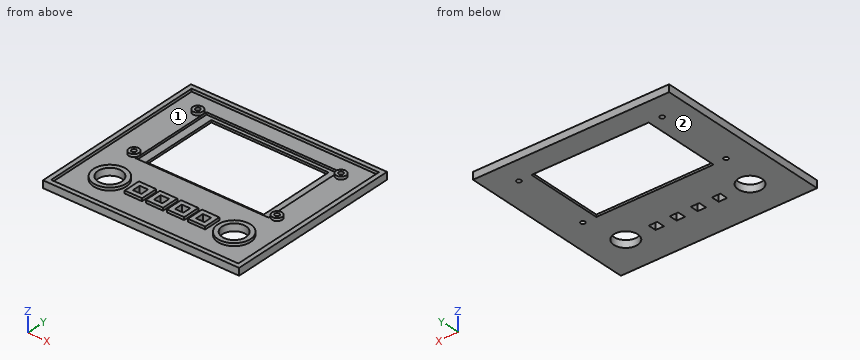
```python
from build123d import *

# Parameters (mm, degrees)
SKETCH1_W           = 139.7
SKETCH1_H           = 127
SKETCH1_R           = 8.5
SKETCH1_W_2         = 6
SKETCH1_H_2         = 5.8
SKETCH1_W_3         = 83.52
SKETCH1_H_3         = 55.68
BOSS_EXTRUDE1_DEPTH = 5.1375
SKETCH2_W           = 94.57
SKETCH2_H           = 60.88
SKETCH2_W_2         = 83.52
SKETCH2_H_2         = 55.68
CUT_EXTRUDE1_DEPTH  = 3.55
SKETCH3_R           = 1.6
SKETCH3_R_2         = 1.6002
CUT_EXTRUDE2_DEPTH  = 10
SKETCH4_W           = 133.35
SKETCH4_H           = 120.65
SKETCH4_R           = 3.6
SKETCH4_R_2         = 3.6002
SKETCH4_R_3         = 11.675
SKETCH4_W_2         = 12.35
SKETCH4_H_2         = 12.15
SKETCH4_W_3         = 94.57
SKETCH4_H_3         = 60.88
CUT_EXTRUDE3_DEPTH  = 1.9625


with BuildPart() as part:
    # Sketch1 → Boss-Extrude1 (new body)
    with BuildSketch(Plane.XY):
        with Locations((-0.265452364, -19.000597583)):
            Rectangle(SKETCH1_W, SKETCH1_H)
        with Locations((44.004207636, -55.869967583)):
            Circle(SKETCH1_R, mode=Mode.SUBTRACT)
        with Locations((-44.535112364, -55.869967583)):
            Circle(SKETCH1_R, mode=Mode.SUBTRACT)
        with Locations((-7.765452364, -55.869967583)):
            Rectangle(SKETCH1_W_2, SKETCH1_H_2, mode=Mode.SUBTRACT)
        Rectangle(SKETCH1_W_3, SKETCH1_H_3, mode=Mode.SUBTRACT)
        with Locations((-22.765452364, -55.869967583)):
            Rectangle(SKETCH1_W_2, SKETCH1_H_2, mode=Mode.SUBTRACT)
        with Locations((7.234547636, -55.869967583)):
            Rectangle(SKETCH1_W_2, SKETCH1_H_2, mode=Mode.SUBTRACT)
        with Locations((22.234547636, -55.869967583)):
            Rectangle(SKETCH1_W_2, SKETCH1_H_2, mode=Mode.SUBTRACT)
    extrude(amount=BOSS_EXTRUDE1_DEPTH)

    # Sketch2 → Cut-Extrude1 (cut)
    with BuildSketch(Plane.XY.offset(5.1375)):
        Rectangle(SKETCH2_W, SKETCH2_H)
        Rectangle(SKETCH2_W_2, SKETCH2_H_2, mode=Mode.SUBTRACT)
    extrude(amount=-CUT_EXTRUDE1_DEPTH, mode=Mode.SUBTRACT)

    # Sketch3 → Cut-Extrude2 (cut)
    with BuildSketch(Plane.XY.offset(5.1375)):
        with Locations((51.005027636, -27.450347583)):
            Circle(SKETCH3_R)
        with Locations((-51.034972364, 27.449652417)):
            Circle(SKETCH3_R)
        with Locations((51.005027636, 27.449652417)):
            Circle(SKETCH3_R)
        with Locations((-51.034972364, -27.449907583)):
            Circle(SKETCH3_R_2)
    extrude(amount=-CUT_EXTRUDE2_DEPTH, mode=Mode.SUBTRACT)

    # Sketch4 → Cut-Extrude3 (cut)
    with BuildSketch(Plane.XY.offset(5.1375)):
        with Locations((-0.265452364, -19.000597583)):
            Rectangle(SKETCH4_W, SKETCH4_H)
        with Locations((51.005027636, -27.450347583)):
            Circle(SKETCH4_R, mode=Mode.SUBTRACT)
        with Locations((-51.034972364, -27.449907583)):
            Circle(SKETCH4_R_2, mode=Mode.SUBTRACT)
        with Locations((-51.034972364, 27.449652417)):
            Circle(SKETCH4_R, mode=Mode.SUBTRACT)
        with Locations((51.005027636, 27.449652417)):
            Circle(SKETCH4_R, mode=Mode.SUBTRACT)
        with Locations((-44.535112364, -55.869967583)):
            Circle(SKETCH4_R_3, mode=Mode.SUBTRACT)
        with Locations((44.004207636, -55.869967583)):
            Circle(SKETCH4_R_3, mode=Mode.SUBTRACT)
        with Locations((22.234547636, -55.869967583)):
            Rectangle(SKETCH4_W_2, SKETCH4_H_2, mode=Mode.SUBTRACT)
        with Locations((-7.765452364, -55.869967583)):
            Rectangle(SKETCH4_W_2, SKETCH4_H_2, mode=Mode.SUBTRACT)
        with Locations((-22.765452364, -55.869967583)):
            Rectangle(SKETCH4_W_2, SKETCH4_H_2, mode=Mode.SUBTRACT)
        with Locations((7.234547636, -55.869967583)):
            Rectangle(SKETCH4_W_2, SKETCH4_H_2, mode=Mode.SUBTRACT)
        Rectangle(SKETCH4_W_3, SKETCH4_H_3, mode=Mode.SUBTRACT)
    extrude(amount=-CUT_EXTRUDE3_DEPTH, mode=Mode.SUBTRACT)


solid = part.part
```
Check sheet for the modelled part. Datum: model origin and axes. Units: mm. Face numbers are marked on the shaded views. Round coordinates to 2 decimals unless told otherwise and drop trailing zeros. Loops run counter-clockwise (first coordinate to the right, second up) from the corner with the lowest first, then second, coordinate; pieces in that order, holes last. Notation, with made-up numbers: (-17, 69) - (35, 69) arc R23 cw to (35, 92) - close; hole circle Ø5 at (-31, 54.25). An arc over 180 degrees is marked (long way). Answer as a JSON object with one key per item and string values. Group by question number.
Q1. Sectioned sample at B-B, the plane y = 22. Enter the section's corners in (x, z) (1 decimal), plus the area to 3 significant figures.
Q2. Sectioned sample at D-D, the plane x = 57.5. Enter the section's corners in (y, z) (1 decimal).
Q3. Sectioned sample at A-A, the plane x = -8. Enter the section's corners in (y, z) (1 decimal).
Q4. Mould release check, pull along Y, two halves, no side actions. Record for the marked faces 1 and 2: released by +Y, released by -Y, zero draft, split by the parting line, or undercut.
Q5. Scan lines: line 1 along Y through (x, z) = (7.5, 1.9); line 2 along Y through (x, z) = (2, 0.45); line 3 along Y through (x, z) = (17, 3.5). Record each from-to range of solid material in increasing order. Write a range as [from, to].
Q6. Sectioned sample at C-C, the plane z = 2.4. Count the separate pieces of the cut face and the enclosed holes in it, plus the area to 3 significant figures.
Solution:
{
 "1": {"outline": "(-70.1, 0) - (-41.8, 0) - (-41.8, 1.6) - (-47.3, 1.6) - (-47.3, 3.2) - (-66.9, 3.2) - (-66.9, 5.1) - (-70.1, 5.1) - close; (41.8, 0) - (69.6, 0) - (69.6, 5.1) - (66.4, 5.1) - (66.4, 3.2) - (47.3, 3.2) - (47.3, 1.6) - (41.8, 1.6) - close", "area": "173 mm²"},
 "2": {"outline": "(-82.5, 0) - (44.5, 0) - (44.5, 5.1) - (41.3, 5.1) - (41.3, 3.2) - (-79.3, 3.2) - (-79.3, 5.1) - (-82.5, 5.1) - close"},
 "3": {"outline": "(-82.5, 0) - (-58.8, 0) - (-58.8, 5.1) - (-61.9, 5.1) - (-61.9, 3.2) - (-79.3, 3.2) - (-79.3, 5.1) - (-82.5, 5.1) - close; (-53, 0) - (-27.8, 0) - (-27.8, 1.6) - (-30.4, 1.6) - (-30.4, 3.2) - (-49.8, 3.2) - (-49.8, 5.1) - (-53, 5.1) - close; (27.8, 0) - (44.5, 0) - (44.5, 5.1) - (41.3, 5.1) - (41.3, 3.2) - (30.4, 3.2) - (30.4, 1.6) - (27.8, 1.6) - close"},
 "4": {"face 1": "undercut", "face 2": "zero draft"},
 "5": {"line 1": "y = [-82.5, -58.77], [-52.97, -30.44], [30.44, 44.5]", "line 2": "y = [-82.5, -27.84], [27.84, 44.5]", "line 3": "y = [-82.5, -79.33], [-61.94, -49.79], [41.32, 44.5]"},
 "6": {"separate pieces": "1", "enclosed holes": "11", "area": "11,400 mm²"}
}
